from build123d import *

# Parameters (mm, degrees)
F0_W     = 133.35
F0_H     = 260.35
F1_DEPTH = 3.175
F2_W     = 12.7
F2_H     = 12.7
F3_DEPTH = 50.8
F4_R     = 1.778
F5_DEPTH = 101.6
F6_R     = 5.08
F7_R     = 7.62


with BuildPart() as f1:
    # F0 (on Top) → F1 (new body)
    with BuildSketch(Plane.XY):
        with Locations((5.6592430919, 17.5170571296)):
            Rectangle(F0_W, F0_H)
    extrude(amount=F1_DEPTH)

    # F2 (on Top) → F3 (join)
    with BuildSketch(Plane.XY):
        with Locations((-44.7109719574, 133.5352105856)):
            Rectangle(F2_W, F2_H)
        with Locations((55.8016305625, 133.2016480923)):
            Rectangle(F2_W, F2_H)
        with Locations((55.8016305625, -97.5674582481)):
            Rectangle(F2_W, F2_H)
        with Locations((-45.7438980997, -98.3642829418)):
            Rectangle(F2_W, F2_H)
        with Locations((57.053201443, 18.1187247694)):
            Rectangle(F2_W, F2_H)
        with Locations((-45.0445456266, 18.4522984385)):
            Rectangle(F2_W, F2_H)
    extrude(amount=F3_DEPTH)

    # F4 (on Top) → F5 (cut)
    with BuildSketch(Plane.XY):
        with Locations((-44.9716448784, 133.486032486)):
            Circle(F4_R)
        with Locations((55.8261945844, 133.486032486)):
            Circle(F4_R)
        with Locations((-45.3700572252, 18.3454081416)):
            Circle(F4_R)
        with Locations((57.4198365211, 17.9469976574)):
            Circle(F4_R)
        with Locations((-45.3700572252, -98.3888506889)):
            Circle(F4_R)
        with Locations((55.8261945844, -98.3888506889)):
            Circle(F4_R)
    extrude(amount=F5_DEPTH, mode=Mode.SUBTRACT)

    # F6
    f6_edges = [f1.edges().sort_by_distance(p)[0] for p in [
        (-38.360972, 127.185211, 26.9875),
        (-38.694546, 24.802298, 26.9875),
        (-38.694546, 12.102298, 26.9875),
        (-39.393898, -92.014283, 26.9875),
        (49.451631, 126.851648, 26.9875),
        (50.703201, 24.468725, 26.9875),
        (49.451631, -91.217458, 26.9875),
        (50.703201, 11.768725, 26.9875),
    ]]
    fillet(f6_edges, radius=F6_R)

    # F7
    f7_edges = [f1.edges().sort_by_distance(p)[0] for p in [
        (-47.250972, 127.185211, 3.175),
        (50.939528, 128.339546, 3.175),
        (-40.182443, 13.590196, 3.175),
        (52.191099, 13.256622, 3.175),
        (-39.393898, -100.904283, 3.175),
        (49.451631, -100.107458, 3.175),
    ]]
    fillet(f7_edges, radius=F7_R)


solid = f1.part
The model under review builds one solid part; all positions refer to its coordinate system, in mm. A direction names the side the tool comes from. Round coordinates to 2 decimals unless told otherwise and drop trailing zeros. Write each loop counter-clockwise with the first axis right and the second up, starting at its lowest first coordinate (ties: lowest second). Pieces come first, ordered by that corner, then holes. Notation, with made-up numbers: (-37, -0.75) - (-14, -0.75) arc R13 ccw to (-14, 20.25) - close; hole circle Ø5 at (40.25, -38). An arc over 180 degrees is marked (long way). One line per item, written item: value. Start each with the question number.
1. Clearance check with flat-ended pins moving along their axes: P1, Ø3, axis at y = 18, z = 21, coming from the +X side; P2, Ø2.5, axis at x = 57.5, z = 28.5, coming from the +Y side; P3, Ø2, axis at x = 55.83, y = -98.39, coming from the -Z side; P4, Ø14, axis at y = 21, z = 38.5, coming from the -X side. State where each tip first meets the part, or that it passes through.
2. The part is to be moulded in two halves that separate along Y. For faces 6 (the face through (58.39, 124.56, 5.35)), 7 (the face through (-47, 127.185, 31)), 8 (the face through (-38.361, 136, 31)), say which applies: released by +Y, released by -Y, zero draft, split by the parting line, or undercut.
3. Consider section A-A on z = 7.5. State how many separate pieces and enclosed holes the cut face has, and give its area (3 significant figures).
4. Consider section C-C on x = -3. Write out the cut boundary in (y, z) (3 decimals), and give its area (3 significant figures).
5. Machinability: for faces 1 (the face through (-47.64, 27.09, 5.35)), 2 (the face through (-36.403, 18.47, 5.348)), 3 (the face through (-52.094, -97, 27)), 4 (the face through (-47.531, 9.811, 5.348)), 5 (the face through (-39.89, 128.63, 31.08)), which of the approach directions +Z, -Z, +X, -X, +Y, -Y give a long, thin tool a straight path to every point of the face, cutting with its end or side? Answer none if there is none.
6. To check wall thickness, follow L1, parallel to Y at x = -48, z = 33; L2, parallel to X at y = 133, z = 39; L3, parallel to Z at x = -25, y = 91 (3 decimals). State the ranges of each line that lie inside material, in increasing order. Write a range as from..to.
7. Consider section B-B on y = 56. Write out the cut boundary in (x, z) (3 decimals).
Checks:
1. P1: stops at x = 63.4
1. P2: stops at y = 139.55
1. P3: passes through
1. P4: stops at x = -51.39
2. face 6: undercut
2. face 7: undercut
2. face 8: zero draft
3. separate pieces: 6
3. enclosed holes: 6
3. area: 988 mm^2
4. outline: (-112.658, 0) - (147.692, 0) - (147.692, 3.175) - (-112.658, 3.175) - close
4. area: 827 mm^2
5. face 1: +Z, +X, -X
5. face 2: +Z, -Y
5. face 3: +Z, -X, +Y, -Y
5. face 4: +Z, -X
5. face 5: +Z
6. L1: y = -104.71..-92.01, 12.1..24.8, 127.19..139.89
6. L2: x = -51.06..-46.68, -43.26..-38.36, 49.45..54.12, 57.54..62.15
6. L3: z = 0..3.175
7. outline: (-61.016, 0) - (72.334, 0) - (72.334, 3.175) - (-61.016, 3.175) - close
